from build123d import *

# Parameters (mm, degrees)
CHAMFER1_SIZE      = 0.5
CUT_EXTRUDE1_DEPTH = 10
EXTRUDE1_DEPTH     = 2.2
EXTRUDE2_DEPTH     = 2.2


with BuildPart() as part:
    # Sketch1 → Revolve1 (revolve)
    with BuildSketch(Plane(origin=(0, 0, 0), x_dir=(1, 0, 0), z_dir=(0, 1, 0))):
        Polygon((0, -57.7), (-7, -57.7), (-7, -56.2), (-4, -56.2), (-4, -19.947651257), (-4, -1.2), (-3.5, -1.2), (-3.5, 0), (-4, 0), (-4, 1.3), (0, 1.3), align=None)
    revolve(axis=Axis((0, 0, -49.376724138), (0, 0, 1)))

    # Chamfer1
    chamfer1_edges = [part.edges().sort_by_distance(p)[0] for p in [
        (4, 0, -1.3),
        (7, 0, 57.7),
    ]]
    chamfer(chamfer1_edges, length=CHAMFER1_SIZE)

    # Sketch2 → Cut-Extrude1 (cut)
    with BuildSketch(Plane(origin=(0, 0, 0), x_dir=(1, 0, 0), z_dir=(0, 1, 0))):
        with BuildLine():
            Line((-1.5, -14.2), (-1.5, -31.2))
            ThreePointArc((-1.5, -31.2), (0, -32.7), (1.5, -31.2))
            Line((1.5, -31.2), (1.5, -14.2))
            ThreePointArc((1.5, -14.2), (0, -12.7), (-1.5, -14.2))
        make_face()
        with BuildLine():
            Line((-1.5, -46.7), (-1.5, -53.7))
            ThreePointArc((-1.5, -53.7), (0, -55.2), (1.5, -53.7))
            Line((1.5, -53.7), (1.5, -46.7))
            ThreePointArc((1.5, -46.7), (0, -45.2), (-1.5, -46.7))
        make_face()
    extrude(amount=CUT_EXTRUDE1_DEPTH, mode=Mode.SUBTRACT)

    # Sketch3 → Extrude1 (add)
    with BuildSketch(Plane(origin=(0, 0, 0), x_dir=(1, 0, 0), z_dir=(0, 1, 0))):
        with BuildLine():
            Line((1.5, -31.2), (1.5, -14.2))
            ThreePointArc((1.5, -14.2), (0, -12.7), (-1.5, -14.2))
            Line((-1.5, -14.2), (-1.5, -31.2))
            ThreePointArc((-1.5, -31.2), (0, -32.7), (1.5, -31.2))
        make_face()
    extrude(amount=EXTRUDE1_DEPTH)

    # Sketch4 → Extrude2 (add)
    with BuildSketch(Plane(origin=(0, 0, 0), x_dir=(1, 0, 0), z_dir=(0, 1, 0))):
        with BuildLine():
            Line((-1.5, -46.7), (-1.5, -53.7))
            ThreePointArc((-1.5, -53.7), (0, -55.2), (1.5, -53.7))
            Line((1.5, -53.7), (1.5, -46.7))
            ThreePointArc((1.5, -46.7), (0, -45.2), (-1.5, -46.7))
        make_face()
    extrude(amount=EXTRUDE2_DEPTH)


solid = part.part
Geometry check sheet. Reference: the model listing, model coordinates, mm. A direction names the side the tool comes from. Round coordinates to 2 decimals unless told otherwise and drop trailing zeros. Order: outer loops, then holes, each group sorted by start corner. A loop starts at its lowest first (then second) coordinate and runs counter-clockwise, first axis right, second up. Notation, with made-up numbers: M 65.5,41.25 L 122.5,41.25 A22 ccw 122.5,50.25 Z; hole C -11,2 d4. An arc over 180 degrees is marked long. Answer in a Markdown table with one row per item. Add a question column.
Item 1: Sectioned sample at D-D, the plane z = 37.5. Enter the section's corners in (x, y).
Item 2: Material ranges on L1, parallel to Z at x = -1.75, y = 4; L2, parallel to X at y = -0.25, z = 18; L3, parallel to Z at x = -2.5, y = 2.75, recorded low to high. Write a range as [from, to].
Item 3: Set-up check for faces 4 (the face through (0, 0, -1.3)), 5 (the face through (0, 2.2, 23)), 6 (the face through (0, 0, 57.7)), 7 (the face through (-2.15, -3.373, 29.085)), 8 (the face through (-3.233, 1.341, 0.592)): record each of +Z, -Z, +X, -X, +Y, -Y from which the full face is reachable in a straight line by a thin tool's end or side.
Item 4: Sectioned sample at C-C, the plane z = 50.5. Enter the section's corners in (x, y).
Item 5: Sectioned sample at A-A, the plane y = 0. Enter the section's corners in (x, z).
Item 6: Draft check along Z on faces 1 (the face through (-3, 3, 56.2)), 2 (the face through (0, 3.1, 12.7)), 3 (the face through (0.867, 3.905, -0.406)). Enter one of: released by +Z, released by -Z, zero draft, split by the parting line, or undercut.
Item 7: Sectioned sample at B-B, the plane x = 0. Enter the section's corners in (y, z).
Item 8: Depth check by flat-ended pin: pin 1 Ø6 at (y, z) = (3.5, 13) entering from +X; pin 2 Ø2 at (x, z) = (3.5, 37.5) entering from -Y; pin 3 Ø8 at (x, y) = (2.5, -4) entering from -Z; pin 4 Ø4 at (x, z) = (1.5, 31) entering from +Y. Enter the tip coordinate at first touch or a pass-through.
Filled in:
| question | item | result |
|---|---|---|
| 1 | outline | C 0,0 d8 |
| 2 | L1 | z = [56.2, 57.7] |
| 2 | L2 | x = [-3.99, 3.99] |
| 2 | L3 | z = [-1.08, 0], [1.2, 57.7] |
| 3 | face 4 | -Z, +X, -X, +Y, -Y |
| 3 | face 5 | +Y |
| 3 | face 6 | +Z, +X, -X, +Y, -Y |
| 3 | face 7 | -Z |
| 3 | face 8 | none |
| 4 | outline | M -1.5,2.2 L -1.5,3.71 A4 ccw long 1.5,3.71 L 1.5,2.2 Z |
| 5 | outline | M -7,56.2 L -4,56.2 L -4,1.2 L -3.5,1.2 L -3.5,0 L -4,0 L -4,-0.8 L -3.5,-1.3 L 3.5,-1.3 L 4,-0.8 L 4,0 L 3.5,0 L 3.5,1.2 L 4,1.2 L 4,56.2 L 7,56.2 L 7,57.2 L 6.5,57.7 L -6.5,57.7 L -7,57.2 Z |
| 6 | face 1 | released by -Z |
| 6 | face 2 | undercut |
| 6 | face 3 | zero draft |
| 7 | outline | M -7,56.2 L -4,56.2 L -4,1.2 L -3.5,1.2 L -3.5,0 L -4,0 L -4,-0.8 L -3.5,-1.3 L 3.5,-1.3 L 4,-0.8 L 4,0 L 3.5,0 L 3.5,1.2 L 4,1.2 L 4,12.7 L 2.2,12.7 L 2.2,32.7 L 4,32.7 L 4,45.2 L 2.2,45.2 L 2.2,55.2 L 4,55.2 L 4,56.2 L 7,56.2 L 7,57.2 L 6.5,57.7 L -6.5,57.7 L -7,57.2 Z |
| 8 | pin 1 | stops at x = 3.97 |
| 8 | pin 2 | stops at y = -3.12 |
| 8 | pin 3 | stops at z = -1.3 |
| 8 | pin 4 | stops at y = 3.98 |
